```python
from build123d import *

# Parameters (mm, degrees)
BOSS_EXTRUDE2_DEPTH = 55
SKETCH8_R           = 7
CUT_EXTRUDE2_DEPTH  = 56
CUT_EXTRUDE3_DEPTH  = 25
CUT_EXTRUDE4_DEPTH  = 20


with BuildPart() as part:
    # Sketch7 → Boss-Extrude2 (new body)
    with BuildSketch(Plane.XY):
        Polygon((0, 0), (80, 0), (80, 25), (50, 25), (50, 12), (25, 12), (25, 35), (12.5, 60), (0, 35), align=None)
    extrude(amount=BOSS_EXTRUDE2_DEPTH)

    # Sketch8 → Cut-Extrude2 (cut, through all)
    with BuildSketch(Plane.XY.offset(55)):
        with Locations((12.5, 25)):
            Circle(SKETCH8_R)
    extrude(amount=-CUT_EXTRUDE2_DEPTH, mode=Mode.SUBTRACT)

    # Sketch10 → Cut-Extrude3 (cut)
    with BuildSketch(Plane.XY.offset(40)):
        Polygon((3.5, 42), (21.5, 42), (12.5, 60), align=None)
    extrude(amount=-CUT_EXTRUDE3_DEPTH, mode=Mode.SUBTRACT)

    # Sketch11 → Cut-Extrude4 (cut)
    with BuildSketch(Plane(origin=(80, 0, 0), x_dir=(0, 0, -1), z_dir=(1, 0, 0))):
        Polygon((-55, 8), (-15, 25), (-55, 25), align=None)
    extrude(amount=-CUT_EXTRUDE4_DEPTH, mode=Mode.SUBTRACT)


solid = part.part
```
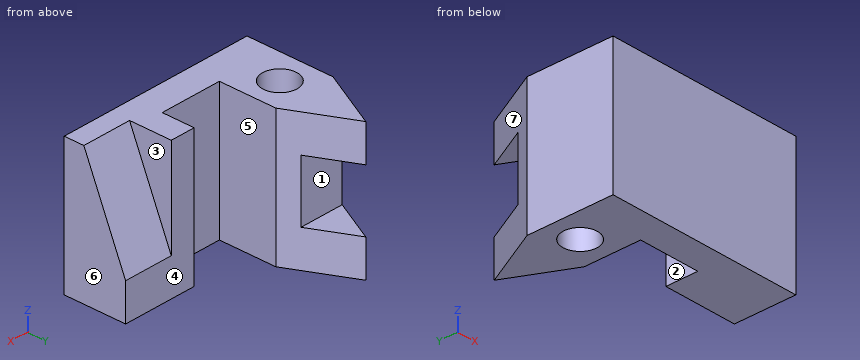
Geometry check sheet. Reference: the model listing, model coordinates, mm. Face numbers are marked on the shaded views. A direction names the side the tool comes from. Coordinates: 2 decimals unless noted, no trailing zeros. Write each loop counter-clockwise with the first axis right and the second up, starting at its lowest first coordinate (ties: lowest second). Pieces come first, ordered by that corner, then holes. Notation, with made-up numbers: M -25,29.5 L 5,29.5 A19 ccw 5,43.5 Z; hole C -36.75,-23.5 d1. An arc over 180 degrees is marked long. Use one line per item in the form item = value. Start each with the question number.
1) Section check D-D on y = 37. Enter the section's corners in (x, z).
2) Section check C-C on z = 20. Enter the section's corners in (x, y) (3 decimals), and give its area (3 significant figures).
3) Thickness scan on probe 1 along X at (y, z) = (17, 25); probe 2 along Y at (x, z) = (12.5, 21.5); probe 3 along Y at (x, z) = (36.5, 45.5). Record the ranges inside material, lowest first. Write a range as from..to.
4) Set-up check for the marked faces 1, 2, 3 and 4: record each of +Z, -Z, +X, -X, +Y, -Y from which the full face is reachable in a straight line by a thin tool's end or side.
5) Section check A-A on y = 22. Enter the section's corners in (x, z).
6) Go/stop test with flat-tipped pins: pin 1 Ø1.5 at (y, z) = (39, 18.5) entering from +X (3 decimals); pin 2 Ø7.5 at (x, z) = (32.5, 28) entering from +Y; pin 3 Ø10 at (y, z) = (53, 34) entering from -X; pin 4 Ø5.5 at (x, z) = (12, 32.5) entering from +Y. Record where each tip stops, or that it passes through.
7) Release check for a two-part mould opening along X. For the marked faces 5, 6 and 7 record: pulls with the +X half, pulls with the -X half, needs draft (parallel to the pull), parting line crosses it, or undercut.
8) Section check B-B on x = 15. Enter the section's corners in (y, z), and give its area (3 significant figures).
Responses:
q1.outline = M 1,0 L 24,0 L 24,55 L 1,55 Z
q2.outline = M 0,0 L 80,0 L 80,22.875 L 60,22.875 L 60,25 L 50,25 L 50,12 L 25,12 L 25,35 L 21.5,42 L 3.5,42 L 0,35 Z; hole C 12.5,25 d14
q2.area = 1,880 mm2
q3.probe_1 = 0..25, 50..80
q3.probe_2 = 0..18, 32..42
q3.probe_3 = 0..12
q4.face_1 = +X, -X, +Y
q4.face_2 = +Z, -Z, +Y
q4.face_3 = +Z, +X, +Y
q4.face_4 = +Z, -Z, +X, +Y
q5.outline = M 0,0 L 6.18,0 L 6.18,55 L 0,55 Z; M 18.82,0 L 25,0 L 25,55 L 18.82,55 Z; M 50,0 L 80,0 L 80,22.06 L 60,22.06 L 60,55 L 50,55 Z
q6.pin_1 = 23.375
q6.pin_2 = 12
q6.pin_3 = through
q6.pin_4 = 42
q7.face_5 = undercut
q7.face_6 = pulls with the +X half
q7.face_7 = pulls with the -X half
q8.outline = M 0,0 L 18.46,0 L 18.46,55 L 0,55 Z; M 31.54,0 L 55,0 L 55,15 L 42,15 L 42,40 L 55,40 L 55,55 L 31.54,55 Z
q8.area = 1,980 mm2
